Check sheet for the modelled part. Datum: model origin and axes. Units: mm. Face numbers are marked on the shaded views. A direction names the side the tool comes from. Round coordinates to 2 decimals unless told otherwise and drop trailing zeros.
from build123d import *

# Parameters (mm, degrees)
F0_R     = 6
F2_DEPTH = 13
F2_TAPER = 1
F3_DEPTH = 12
F5_R     = 0.7494732789
F6_DEPTH = 13
F6_TAPER = -2


with BuildPart() as f2:
    # F0 (on Top) → F2 (new body)
    with BuildSketch(Plane.XY):
        Circle(F0_R)
    extrude(amount=F2_DEPTH, taper=F2_TAPER)

    # F1 (on Top) → F3 (cut)
    with BuildSketch(Plane.XY):
        with BuildLine():
            ThreePointArc((-1.46, -2.6207632476), (1.5198684154, -2.5865034313), (3, 0))
            ThreePointArc((3, 0), (1.5198684154, 2.5865034313), (-1.46, 2.6207632476))
            Line((-1.46, 2.6207632476), (-1.46, 0))
            Line((-1.46, 0), (-1.46, -2.6207632476))
        make_face()
    extrude(amount=F3_DEPTH, mode=Mode.SUBTRACT)

    # F5 (on face) → F6 (cut)
    with BuildSketch(Plane(origin=(0, 0, 0), x_dir=(1, 0, 0), z_dir=(0, 0, -1))):
        with Locations((0, 6.5)):
            Circle(F5_R)
        with Locations((-2.2231309316, 6.1080020351)):
            Circle(F5_R)
        with Locations((-4.178119463, 4.9792888803)):
            Circle(F5_R)
        with Locations((-5.6291651246, 3.25)):
            Circle(F5_R)
        with Locations((-6.4012503946, 1.1287131548)):
            Circle(F5_R)
        with Locations((-6.4012503946, -1.1287131548)):
            Circle(F5_R)
        with Locations((-5.6291651246, -3.25)):
            Circle(F5_R)
        with Locations((-4.178119463, -4.9792888803)):
            Circle(F5_R)
        with Locations((-2.2231309316, -6.1080020351)):
            Circle(F5_R)
        with Locations((0, -6.5)):
            Circle(F5_R)
        with Locations((2.2231309316, -6.1080020351)):
            Circle(F5_R)
        with Locations((4.178119463, -4.9792888803)):
            Circle(F5_R)
        with Locations((5.6291651246, -3.25)):
            Circle(F5_R)
        with Locations((6.4012503946, -1.1287131548)):
            Circle(F5_R)
        with Locations((6.4012503946, 1.1287131548)):
            Circle(F5_R)
        with Locations((5.6291651246, 3.25)):
            Circle(F5_R)
        with Locations((4.178119463, 4.9792888803)):
            Circle(F5_R)
        with Locations((2.2231309316, 6.1080020351)):
            Circle(F5_R)
    extrude(amount=-F6_DEPTH, taper=F6_TAPER, mode=Mode.SUBTRACT)


solid = f2.part
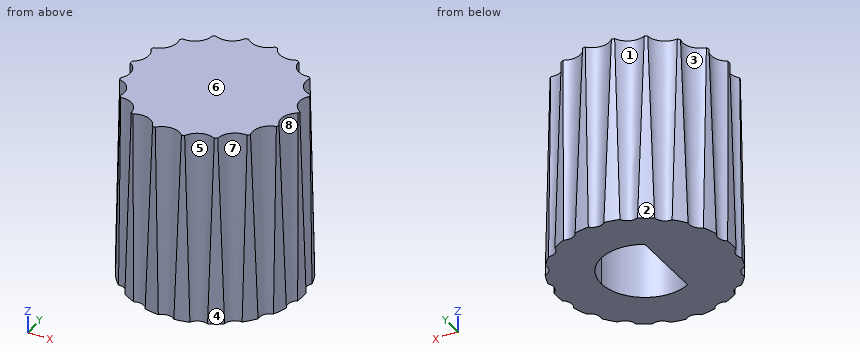
1. Set-up check for the marked faces 1, 2, 3, 4 and 5: record each of +Z, -Z, +X, -X, +Y, -Y from which the full face is reachable in a straight line by a thin tool's end or side.
2. Release check for a two-part mould opening along Y. For the marked faces 6, 7 and 8 record: released by +Y, released by -Y, zero draft, split by the parting line, or undercut.
3. Go/stop test with flat-tipped pins: pin 1 (1.5 mm diameter, centred on y = -3.5, z = 8, fed in from +X); pin 2 (2.5 mm diameter, centred on y = -1, z = 7.5, fed in from +X); pin 3 (2 mm diameter, centred on y = -2, z = 4.5, fed in from +X); pin 4 (4 mm diameter, centred on x = 4, y = -4.5, fed in from -Z). Record where each tip stops, or that it passes through.
4. Scan lines: line 1 along X through (y, z) = (2.5, 8); line 2 along Y through (x, z) = (-1.25, 8); line 3 along Y through (x, z) = (0.5, 4.75). Record each from-to range of solid material in increasing order.
Computed values:
1. face 1: +Z, +Y
1. face 2: +Z, -X, +Y
1. face 3: +Z, -X
1. face 4: +Z, +X, -Y
1. face 5: +Z, -Y
2. face 6: zero draft
2. face 7: released by -Y
2. face 8: undercut
3. pin 1: stops at x = 4.73
3. pin 2: stops at x = 5.88
3. pin 3: stops at x = 5.7
3. pin 4: stops at z = 0
4. line 1: x = -4.92 to -1.46, 1.66 to 4.92
4. line 2: y = -5.73 to -2.73, 2.73 to 5.73
4. line 3: y = -5.73 to -2.96, 2.96 to 5.73
